```python
from build123d import *

# Parameters (mm, degrees)
ESQUISSE2_R        = 14.2
BOSS_EXTRU_8_DEPTH = 6.48
BOSS_EXTRU_9_DEPTH = 2.1


with BuildPart() as part:
    # Esquisse2 → Boss.-Extru.8 (new body)
    with BuildSketch(Plane.XY):
        Circle(ESQUISSE2_R)
        with BuildLine():
            Line((1.483428969, -2.23993348), (2.953146627, -1.705))
            Line((2.953146627, -1.705), (9.950631889, -5.745))
            ThreePointArc((9.950631889, -5.745), (3.929811447, -10.797068213), (-3.929811447, -10.797068213))
            Line((-3.929811447, -10.797068213), (-1.166288689, -3.204351837))
            Line((-1.166288689, -3.204351837), (0.339010323, -2.656467803))
            Line((0.339010323, -2.656467803), (-0.017447021, -1.677109299))
            Line((-0.017447021, -1.677109299), (-0.056805783, -1.568971989))
            ThreePointArc((-0.056805783, -1.568971989), (-1.2591971, -0.93772206), (-1.519465743, 0.395125113))
            Line((-1.519465743, 0.395125113), (0.909996763, 1.27937715))
            ThreePointArc((0.909996763, 1.27937715), (1.566031564, 0.111557793), (1.082162789, -1.137463712))
            Line((1.082162789, -1.137463712), (1.126971625, -1.260574976))
            Line((1.126971625, -1.260574976), (1.483428969, -2.23993348))
        make_face(mode=Mode.SUBTRACT)
        with BuildLine():
            Line((-7.385629635, 8.801850651), (-2.191905749, 2.612211551))
            ThreePointArc((-2.191905749, 2.612211551), (-2.953146627, 1.705), (-3.358194438, 0.592140286))
            ThreePointArc((-3.358194438, 0.592140286), (-3.358194438, -0.592140286), (-2.953146627, -1.705))
            Line((-2.953146627, -1.705), (-9.950631889, -5.745))
            ThreePointArc((-9.950631889, -5.745), (-11.315441082, 1.995217561), (-7.385629635, 8.801850651))
        make_face(mode=Mode.SUBTRACT)
        with BuildLine():
            Line((0, 3.41), (0, 11.49))
            ThreePointArc((0, 11.49), (7.912534617, 8.331380194), (11.4747318, 0.592140286))
            Line((11.4747318, 0.592140286), (3.358194438, 0.592140286))
            ThreePointArc((3.358194438, 0.592140286), (2.191905749, 2.612211551), (0, 3.41))
        make_face(mode=Mode.SUBTRACT)
    extrude(amount=BOSS_EXTRU_8_DEPTH)

    # Esquisse6 → Boss.-Extru.9 (add)
    with BuildSketch(Plane.XY.offset(6.48)):
        with BuildLine():
            Line((-1.519465743, 0.395125113), (0.909996763, 1.27937715))
            ThreePointArc((0.909996763, 1.27937715), (1.566031564, 0.111557793), (1.082162789, -1.137463712))
            Line((1.082162789, -1.137463712), (1.483428969, -2.23993348))
            Line((1.483428969, -2.23993348), (2.953146627, -1.705))
            ThreePointArc((2.953146627, -1.705), (-1.166288689, 3.204351837), (-1.166288689, -3.204351837))
            Line((-1.166288689, -3.204351837), (0.339010323, -2.656467803))
            Line((0.339010323, -2.656467803), (-0.056805783, -1.568971989))
            ThreePointArc((-0.056805783, -1.568971989), (-1.2591971, -0.93772206), (-1.519465743, 0.395125113))
        make_face()
    extrude(amount=BOSS_EXTRU_9_DEPTH)


solid = part.part
```
Check sheet for the modelled part. Datum: model origin and axes. Units: mm. A direction names the side the tool comes from. Round coordinates to 2 decimals unless told otherwise and drop trailing zeros. Loops run counter-clockwise (first coordinate to the right, second up) from the corner with the lowest first, then second, coordinate; pieces in that order, holes last. Notation, with made-up numbers: (24, 75.25) - (81, 75.25) arc R22 cw to (81, 86.25) - close; hole circle Ø4 at (48.5, 45). An arc over 180 degrees is marked (long way). Answer as a JSON object with one key per item and string values. Group by question number.
Q1. Sectioned sample at C-C, the plane x = 6.75. Enter the section's corners in (y, z).
Q2. Mould release check, pull along X, two halves, no side actions. Record for faces 3 (the face through (-4.825, 5.75, 3.195)), 4 (the face through (-2.567, -7.054, 3.195)), 5 (the face through (-3, -3, 6.48)), 6 (the face through (-1.85, 14.08, 3.19)): released by +X, released by -X, zero draft, split by the parting line, or undercut.
Q3. Gauge pin test, flat ends, axial feed: P1, Ø4, axis at y = -2.5, z = 1, coming from the -X side; P2, Ø1.5, axis at x = -10, y = 1.5, coming from the +Z side; P3, Ø4, axis at y = -6, z = 5, coming from the -X side (3 decimals); P4, Ø6, axis at x = -9, y = 2, coming from the +Z side. Record the tip position at first contact, or that the pin passes through.
Q4. Sectioned sample at B-B, the plane z = 2. Enter the section's corners in (x, y) (3 decimals), plus the area to 3 significant figures.
Q5. Sectioned sample at A-A, the plane y = 0. Enter the section's corners in (x, z), plus the area to 3 significant figures.
Q6. Scan lines: line 1 along Y through (x, z) = (5.5, 3); line 2 along X through (y, z) = (-2.5, 2.5); line 3 along X through (y, z) = (1.75, 5.75). Record each from-to range of solid material in increasing order. Write a range as [from, to].
Q7. Set-up check for faces 1 (the face through (6.403, -3.697, 3.195)), 2 (the face through (-1, 1, 8.58)): record each of +Z, -Z, +X, -X, +Y, -Y from which the full face is reachable in a straight line by a thin tool's end or side.
Q8. Sectioned sample at D-D, the plane y = -7.75. Enter the section's corners in (x, z).
Solution:
{
 "1": {"outline": "(-12.49, 0) - (-9.3, 0) - (-9.3, 6.48) - (-12.49, 6.48) - close; (-3.9, 0) - (0.59, 0) - (0.59, 6.48) - (-3.9, 6.48) - close; (9.3, 0) - (12.49, 0) - (12.49, 6.48) - (9.3, 6.48) - close"},
 "2": {"face 3": "undercut", "face 4": "undercut", "face 5": "zero draft", "face 6": "split by the parting line"},
 "3": {"P1": "stops at x = -14.19", "P2": "passes through", "P3": "stops at x = -13.625", "P4": "stops at z = 6.48"},
 "4": {"outline": "circle Ø28.4 at (0, 0); hole (-9.951, -5.745) - (-2.953, -1.705) arc R3.41 cw to (-2.192, 2.612) - (-7.386, 8.802) arc R11.49 ccw to start; hole (-3.93, -10.797) arc R11.49 ccw to (9.951, -5.745) - (2.953, -1.705) - (1.483, -2.24) - (1.082, -1.137) arc R1.57 ccw to (0.91, 1.279) - (-1.519, 0.395) arc R1.57 ccw to (-0.057, -1.569) - (0.339, -2.656) - (-1.166, -3.204) - close; hole (0, 3.41) arc R3.41 cw to (3.358, 0.592) - (11.475, 0.592) arc R11.49 ccw to (0, 11.49) - close", "area": "365 mm²"},
 "5": {"outline": "(-14.2, 0) - (-11.49, 0) - (-11.49, 6.48) - (-14.2, 6.48) - close; (-3.41, 0) - (-1.57, 0) - (-1.57, 8.58) - (-3.41, 8.58) - close; (1.57, 0) - (14.2, 0) - (14.2, 6.48) - (3.41, 6.48) - (3.41, 8.58) - (1.57, 8.58) - close", "area": "119 mm²"},
 "6": {"line 1": "y = [-13.09, -10.09], [-3.18, 0.59], [10.09, 13.09]", "line 2": "x = [-13.98, -11.21], [-4.33, 0.28], [4.33, 13.98]", "line 3": "x = [-14.09, -11.36], [-2.93, 2.93], [11.36, 14.09]"},
 "7": {"face 1": "+Z, -Z", "face 2": "+Z, +X, -X, +Y, -Y"},
 "8": {"outline": "(-11.9, 0) - (-2.82, 0) - (-2.82, 6.48) - (-11.9, 6.48) - close; (8.48, 0) - (11.9, 0) - (11.9, 6.48) - (8.48, 6.48) - close"}
}
